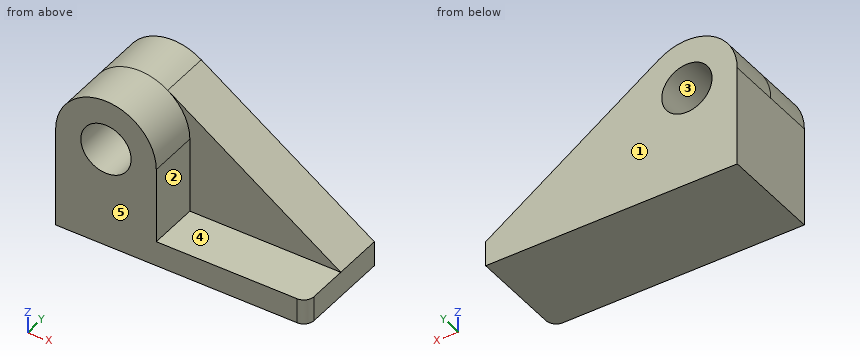
from build123d import *

# Parameters (mm, degrees)
F0_R     = 12.7
F1_DEPTH = 25.4
F2_R     = 12.7
F3_DEPTH = 25.4
F4_DEPTH = 25.4
F5_R     = 5.08


with BuildPart() as f1:
    # F0 (on Front) → F1 (new body)
    with BuildSketch(Plane.XZ):
        with BuildLine():
            Line((64.7399425507, 12.7), (-22.6221843212, 71.8343283417))
            ThreePointArc((-22.6221843212, 71.8343283417), (-48.766316781, 73.2365993129), (-62.2600574493, 50.8))
            Line((-62.2600574493, 50.8), (-62.2600574493, 0))
            Line((-62.2600574493, 0), (64.7399425507, 0))
            Line((64.7399425507, 0), (64.7399425507, 12.7))
        make_face()
        with Locations((-36.8600574493, 50.8)):
            Circle(F0_R, mode=Mode.SUBTRACT)
    extrude(amount=F1_DEPTH)

    # F2 (on face) → F3 (join)
    with BuildSketch(Plane.XZ.offset(25.4)):
        with BuildLine():
            Line((64.7399425507, 0), (64.7399425507, 12.7))
            Line((64.7399425507, 12.7), (-11.4600574493, 12.7))
            Line((-11.4600574493, 12.7), (-11.4600574493, 50.8))
            ThreePointArc((-11.4600574493, 50.8), (-36.8600574493, 76.2), (-62.2600574493, 50.8))
            Line((-62.2600574493, 50.8), (-62.2600574493, 12.7))
            Line((-62.2600574493, 12.7), (-62.2600574493, 0))
            Line((-62.2600574493, 0), (64.7399425507, 0))
        make_face()
        with Locations((-36.8600574493, 50.8)):
            Circle(F2_R, mode=Mode.SUBTRACT)
    extrude(amount=F3_DEPTH)

    # F2 (on face) → F4 (join)
    with BuildSketch(Plane.XZ.offset(25.4)):
        with BuildLine():
            Line((64.7399425507, 0), (64.7399425507, 12.7))
            Line((64.7399425507, 12.7), (-11.4600574493, 12.7))
            Line((-11.4600574493, 12.7), (-11.4600574493, 50.8))
            ThreePointArc((-11.4600574493, 50.8), (-14.4234581364, 62.7062593317), (-22.6221843212, 71.8343283417))
            ThreePointArc((-22.6221843212, 71.8343283417), (-48.766316781, 73.2365993129), (-62.2600574493, 50.8))
            Line((-62.2600574493, 50.8), (-62.2600574493, 12.7))
            Line((-62.2600574493, 12.7), (-62.2600574493, 0))
            Line((-62.2600574493, 0), (64.7399425507, 0))
        make_face()
        with Locations((-36.8600574493, 50.8)):
            Circle(F2_R, mode=Mode.SUBTRACT)
    extrude(amount=F4_DEPTH)

    # F5
    f5_edges = [f1.edges().sort_by_distance(p)[0] for p in [
        (64.739943, -50.8, 6.35),
    ]]
    fillet(f5_edges, radius=F5_R)


solid = f1.part
Geometry check sheet. Reference: the model listing, model coordinates, mm. Face numbers are marked on the shaded views. A direction names the side the tool comes from. Give positions to 0.01 mm unless a question says otherwise; leave off trailing zeros. Order: outer loops, then holes, each group sorted by start corner. A loop starts at its lowest first (then second) coordinate and runs counter-clockwise, first axis right, second up. Notation, with made-up numbers: (20.25, 0) - (68.25, 0) arc R19 ccw to (68.25, 12) - close; hole circle Ø8 at (12, -32.75). An arc over 180 degrees is marked (long way). Use one line per item in the form item = value.
1) Access from +Z, -Z, +X, -X, +Y, -Y to the whole of each face (thin tool, end or side, straight path). Record for the marked faces 1 and 2.
Working result:
face_1 = +Z, -Z, +X, -X, +Y
face_2 = +Z, +X, -Y
2) Draft check along Z on the marked faces 3, 4 and 5. Enter one of: released by +Z, released by -Z, zero draft, split by the parting line, or undercut.
Working result:
face_3 = undercut
face_4 = released by +Z
face_5 = zero draft
3) Sectioned sample at A-A (y = -32). Record the boundary of the cut face in (x, z).
Working result:
outline = (-62.26, 0) - (64.74, 0) - (64.74, 12.7) - (-11.46, 12.7) - (-11.46, 50.8) arc R25.4 ccw to (-62.26, 50.8) - close; hole circle Ø25.4 at (-36.86, 50.8)
4) Material ranges on probe 1 along Y at (x, z) = (-1.5, 37); probe 2 along X at (y, z) = (-22.5, 41.5); probe 3 along Z at (x, y) = (34, -47), recorded low to high. Write a range as from..to.
Working result:
probe_1 = -25.4..0
probe_2 = -62.26..-45.51, -28.21..22.19
probe_3 = 0..12.7
5) Depth check by flat-ended pin: pin 1 Ø20.5 at (x, y) = (24.5, -41.5) entering from +Z; pin 2 Ø2 at (x, y) = (-18, -33) entering from -Z; pin 3 Ø1.5 at (x, y) = (23, -24.5) entering from +Z; pin 4 Ø5 at (x, y) = (-44.5, -22) entering from +Z. Enter the tip coordinate at first touch or a pass-through.
Working result:
pin_1 = 12.7
pin_2 = 0
pin_3 = 41.46
pin_4 = 75.67
6) Sectioned sample at B-B (x = -42). Record the boundary of the cut face in (y, z).
Working result:
outline = (-50.8, 0) - (0, 0) - (0, 39.19) - (-50.8, 39.19) - close; (-50.8, 62.41) - (0, 62.41) - (0, 75.67) - (-50.8, 75.67) - close
7) Sectioned sample at C-C (z = 45). Record the boundary of the cut face in (x, y), and give its area (3 significant figures).
Working result:
outline = (-62.26, -50.8) - (-48.16, -50.8) - (-48.16, 0) - (-62.26, 0) - close; (-25.56, -50.8) - (-11.46, -50.8) - (-11.46, -25.4) - (17.02, -25.4) - (17.02, 0) - (-25.56, 0) - close
area = 2,160 mm^2
8) Sectioned sample at D-D (x = 24.5). Record the boundary of the cut face in (y, z), and give its area (3 significant figures).
Working result:
outline = (-50.8, 0) - (0, 0) - (0, 39.94) - (-25.4, 39.94) - (-25.4, 12.7) - (-50.8, 12.7) - close
area = 1,340 mm^2
